from build123d import *

# Parameters (mm, degrees)
CROQUIS2_R              = 75
CROQUIS2_R_2            = 3.175
CROQUIS2_R_3            = 12.5
SALIENTE_EXTRUIR2_DEPTH = 5


with BuildPart() as part:
    # Croquis2 → Saliente-Extruir2 (new body)
    with BuildSketch(Plane(origin=(0, 0, 0), x_dir=(1, 0, 0), z_dir=(0, 1, 0))):
        Polygon((-164.024069274, 177.568942162), (-164.024069274, -142.431057838), (-164.024069274, -189.256710106), (-164.024069274, -222.426710106), (-79.024069274, -222.426710106), (-9.024069274, -222.426710106), (-9.024069274, -112.958468136), (275.975930726, -112.958468136), (275.975930726, 177.568942162), align=None)
        with Locations(Location((70.975930726, 30.02579809, 0), (0, 0, 270))):
            Circle(CROQUIS2_R, mode=Mode.SUBTRACT)
        with Locations(Location((209.175930726, 30.02579809, 0), (0, 0, 270))):
            Circle(CROQUIS2_R_2, mode=Mode.SUBTRACT)
        with Locations(Location((-67.224069274, 30.02579809, 0), (0, 0, 270))):
            Circle(CROQUIS2_R_2, mode=Mode.SUBTRACT)
        with Locations(Location((70.975930726, 160.02579809, 0), (0, 0, 270))):
            Circle(CROQUIS2_R_2, mode=Mode.SUBTRACT)
        with Locations(Location((-44.024069274, -177.958468136, 0), (0, 0, 270))):
            Circle(CROQUIS2_R_3, mode=Mode.SUBTRACT)
    extrude(amount=SALIENTE_EXTRUIR2_DEPTH)


solid = part.part
The model under review builds one solid part; all positions refer to its coordinate system, in mm. Coordinates: 2 decimals unless noted, no trailing zeros. Loops run counter-clockwise (first coordinate to the right, second up) from the corner with the lowest first, then second, coordinate; pieces in that order, holes last.
(1) Consider section B-B, the plane z = 185. Give the boundary of the cut face in (x, y).
Determined:
outline: (-164.02, 0) - (-54.35, 0) - (-54.35, 5) - (-164.02, 5) - close; (-33.7, 0) - (-9.02, 0) - (-9.02, 5) - (-33.7, 5) - close
(2) Consider section C-C, the plane y = 1.65. Give the boundary of the cut face in (x, z) (3 decimals), plus the area to 3 significant figures.
Determined:
outline: (-164.024, -177.569) - (275.976, -177.569) - (275.976, 112.958) - (-9.024, 112.958) - (-9.024, 222.427) - (-164.024, 222.427) - close; hole circle Ø6.35 at (-67.224, -30.026); hole circle Ø25 at (-44.024, 177.958); hole circle Ø150 at (70.976, -30.026); hole circle Ø6.35 at (70.976, -160.026); hole circle Ø6.35 at (209.176, -30.026)
area: 127,000 mm2
(3) Draft analysis for pull direction X (two halves, no side actions). For faces 1 (the cylindrical face through (-43.47, 2.46, 165.47)), 2 (the flat face through (4, 5, 20)), state which applies: +X half, -X half, draft (parallel to the pull), parting line (faces both ways), or undercut.
Determined:
face 1: undercut
face 2: draft
(4) Insertion check: P1, Ø1, axis at y = 3, z = 122, coming from the +X side. The pin has a flat end and moves straight along its axis. Give the tip position at first contact, or say it passes through.
Determined:
P1: stops at x = -9.02
(5) Wall thickness on L1, parallel to Z at x = 186, y = 3.1; L2, parallel to X at y = 2.6, z = -11; L3, parallel to X at y = 4.4, z = 180: over which ranges is each line inside the solid? List them lowest first.
Determined:
L1: z = -177.57 to 112.96
L2: x = -164.02 to -1.57, 143.52 to 275.98
L3: x = -164.02 to -56.36, -31.69 to -9.02
(6) Consider section A-A, the plane x = 84. Give the boundary of the cut face in (y, z), plus the area to 3 significant figures.
Determined:
outline: (0, -177.57) - (5, -177.57) - (5, -103.89) - (0, -103.89) - close; (0, 43.83) - (5, 43.83) - (5, 112.96) - (0, 112.96) - close
area: 714 mm2
